Can you work these out from the model? Positions are in its coordinate system, mm. A direction names the side the tool comes from. Coordinates: 2 decimals unless noted, no trailing zeros. Write each loop counter-clockwise with the first axis right and the second up, starting at its lowest first coordinate (ties: lowest second). Pieces come first, ordered by that corner, then holes. Notation, with made-up numbers: (-16, 22.5) -> (39, 22.5) arc R24 cw to (39, 59.5) -> close; hole circle Ø2 at (-12, 4). An arc over 180 degrees is marked (long way). Answer as CSV lines item,"result". Start each with the question number.
```python
from build123d import *

# Parameters (mm, degrees)
SKETCH_1_R          = 7.5
EXTRUDE_1_DEPTH     = 12
SKETCH_3_R          = 2.5
EXTRUDE_2_DEPTH     = 150
CUT_EXTRUDE_1_REACH = 152.666
SKETCH_2_R          = 3


with BuildPart() as part:
    # 草图1 → 凸台-拉伸1 (new body)
    with BuildSketch(Plane(origin=(0, 0, 0), x_dir=(0, 0, -1), z_dir=(1, 0, 0))):
        Circle(SKETCH_1_R)
    extrude(amount=EXTRUDE_1_DEPTH)

    # 草图3 → 凸台-拉伸2 (add)
    with BuildSketch(Plane(origin=(0, 0, 0), x_dir=(1, 0, 0), z_dir=(0, 1, 0))):
        with Locations(Location((6.065609695, 0, 0), (0, 0, 90))):
            Circle(SKETCH_3_R)
    extrude(amount=EXTRUDE_2_DEPTH)

    # 草图2 → 切除-拉伸1 (cut, up to next)
    with BuildSketch(Plane(origin=(12, 0, 0), x_dir=(0, 0, -1), z_dir=(1, 0, 0)), mode=Mode.PRIVATE) as cut_extrude_1_sk1:
        Circle(SKETCH_2_R)
    cut_extrude_1_tool1 = extrude(cut_extrude_1_sk1.sketch, amount=-CUT_EXTRUDE_1_REACH, mode=Mode.PRIVATE) & part.part
    add(cut_extrude_1_tool1.solids().sort_by_distance((12, 0, 0))[0], mode=Mode.SUBTRACT)


solid = part.part
```
Q1. Imagine slicing it at A-A (z = 0). Write out the boundary of the cut face in (x, y), then the cut area to 4 significant figures.
Q2. Imagine slicing it at B-B (y = 0). Write out the boundary of the cut face in (x, z).
Q3. Imagine slicing it at C-C (y = 49). Write out the boundary of the cut face in (x, z), then the cut area to 3 significant figures.
Q4. If we mould it in two halves opening along Z, with no side actions, what happens to faces 1 (the face through (5.92, -7.32, 1.63)), 2 (the face through (0, 0.1, -3.2)), 3 (the face through (6, 0, 3))? For each: released by +Z, released by -Z, zero draft, split by the parting line, or undercut.
Q5. Which directions (+Z, -Z, +X, -X, +Y, -Y) give clear straight access to the entire face, cutting with the end or side of a thin tool? Please do faces 4 (the face through (3.587, 77.535, 0.325)), 5 (the face through (12, 0.1, -3.2)).
Q6. For pin 1 (2 mm diameter, centred on y = 114, z = 2, fed in from +X); pin 2 (3 mm diameter, centred on x = 5, y = 68, fed in from -Z); pin 3 (2 mm diameter, centred on y = 85.5, z = -2, fed in from -X); pin 4 (5 mm diameter, centred on y = 0, z = 0, fed in from -X), each with a flat end and sliding along its axis, tell me the tip position at first contact or that it passes through.
Q7. I need wall thicknesses on L1, parallel to Y at x = 7.75, z = 0; L2, parallel to Y at x = 8.75, z = -1; L3, parallel to X at y = 76, z = 1.5. Which ranges of each line are inside material? Lowest first, please.
Entries:
1,outline,"(0, -7.5) -> (12, -7.5) -> (12, -3) -> (0, -3) -> close; (0, 3) -> (12, 3) -> (12, 7.5) -> (8.57, 7.5) -> (8.57, 150) -> (3.57, 150) -> (3.57, 7.5) -> (0, 7.5) -> close"
1,area,"820.5 mm2"
2,outline,"(0, -7.5) -> (12, -7.5) -> (12, -3) -> (0, -3) -> close; (0, 3) -> (12, 3) -> (12, 7.5) -> (0, 7.5) -> close"
3,outline,"circle Ø5 at (6.07, 0)"
3,area,"19.6 mm2"
4,face 1,"split by the parting line"
4,face 2,"zero draft"
4,face 3,"undercut"
5,face 4,"+Y"
5,face 5,"+Z, -Z, +X, +Y, -Y"
6,pin 1,"x = 8.36"
6,pin 2,"z = -2.5"
6,pin 3,"x = 3.77"
6,pin 4,"through"
7,L1,"-7.5 to -3, 3 to 150"
7,L2,"-7.43 to -2.83, 2.83 to 7.43"
7,L3,"4.07 to 8.07"
